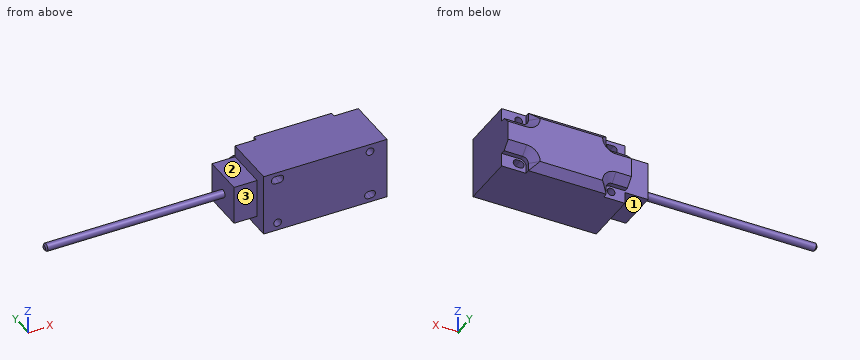
Autodesk Inventor part; units mm, degrees
ref_plane "Work Plane1" through (0, 0, -20) normal (0, 0, 1) x (1, 0, 0)
ref_plane "YZ Plane" through (0, 0, 0) normal (1, 0, 0) x (0, 1, 0)
ref_plane "XZ Plane" through (0, 0, 0) normal (0, 1, 0) x (-1, 0, 0)
sketch "Sketch1" plane through (0, 0, 0) normal (0, 0, 1) x (1, 0, 0)
  line L0 (0, 0) -> (80, 0)
  line L1 (80, 0) -> (80, 43)
  line L2 (80, 43) -> (0, 43)
  line L3 (0, 43) -> (0, 0)
  dimension "d0" = 80
  dimension "d1" = 43
extrude "Extrusion1" add sketch "Sketch1" against normal blind 40
sketch "Sketch2" plane through (0, 43, 0) normal (0, 1, 0) x (1, 0, 0)
  line L0 (80, 0) -> (80, 40)
  circle A0 centre (69, 5) radius 2.5
  arc A1 (7.5, 7.5) -> (7.5, 2.5) centre (7.5, 5) ccw
  arc A2 (10.5, 2.5) -> (10.5, 7.5) centre (10.5, 5) ccw
  line L1 (7.5, 7.5) -> (10.5, 7.5)
  line L2 (10.5, 2.5) -> (7.5, 2.5)
  arc A3 (68, 37.5) -> (68, 32.5) centre (68, 35) ccw
  arc A4 (69.5, 32.5505) -> (70, 37.5) centre (70, 35) ccw
  line L3 (68, 37.5) -> (70, 37.5)
  line L4 (68, 32.5) -> (70, 32.5)
  point P0 (0, 0)
  point P1 (69, 35)
  point P2 (9, 5)
  point P3 (9, 35)
  dimension "d4" = 11
  dimension "d5" = 30
  dimension "d6" = 5
  dimension "d7" = 60
  dimension "d16" = 5
  dimension "d17" = 5
  dimension "d18" = 5
  dimension "d19" = 1.5
  dimension "d20" = 1.5
  dimension "d24" = 5
  dimension "d25" = 5
hole "Hole1" at (69, 43, -5) at (9, 43, -35) direction (0, -1, 0) diameter 5 end through all
extrude "Extrusion2" cut sketch "Sketch2" against normal through all contours L1 A2 L2 A1 | L3 A4 L4 A3
sketch "Sketch3" plane through (0, 43, 0) normal (0, 1, 0) x (1, 0, 0)
  arc A0 (64.25, 35) -> (68, 31.25) centre (68, 35) ccw
  line L0 (64.25, 35) -> (64.25, 40)
  line L1 (68, 31.25) -> (80, 31.25)
  line L2 (64.25, 40) -> (80, 40)
  line L3 (80, 40) -> (80, 31.25)
  line L4 (80, 0) -> (80, 40)
  arc A1 (13.75, 5) -> (10, 8.75) centre (10, 5) ccw
  line L5 (10, 8.75) -> (0, 8.75)
  line L6 (13.75, 5) -> (13.75, 0)
  line L7 (0, 0) -> (80, 0)
  line L8 (0, 0) -> (0, 40)
  line L9 (0, 8.75) -> (0, 0)
  line L10 (0, 0) -> (13.75, 0)
  point P0 (9, 5)
  point P1 (69, 5)
  point P2 (69, 35)
  dimension "d29" = 7.5
  dimension "d34" = 7.5
  dimension "d35" = 1
extrude "Extrusion3" cut sketch "Sketch3" against normal blind 8
ref_plane "Work Plane1" through (0, 0, -20) normal (0, 0, 1) x (1, 0, 0)
mirror "Mirror2" about plane through (0, 0, -20) normal (0, 0, 1) of "Extrusion3"
chamfer "Chamfer1" distance 5 angle 45 14 edges at (39, 43, 0) (39, 43, -40) (5, 43, -8.75) (12.6517, 43, -7.6517) (13.75, 43, -2.5) (12.6517, 43, -32.3483) (5, 43, -31.25) (13.75, 43, -37.5) (74, 43, -31.25) (65.3483, 43, -32.3483) (64.25, 43, -37.5) (74, 43, -8.75) (65.3483, 43, -7.6517) (64.25, 43, -2.5)
sketch "Sketch4" plane through (0, 0, -40) normal (-1, 0, 0) x (0, 0, 1)
  line L0 (7.5, 35) -> (2.5, 35)
  line L1 (7.5, 35) -> (32.5, 35)
  line L2 (32.5, 35) -> (32.5, 8.0021)
  line L3 (32.5, 8.0021) -> (7.5, 8.0021)
  line L4 (7.5, 8.0021) -> (7.5, 35)
  line L5 (7.5, 35) -> (2.5, 35)
  point P0 (40, 0)
extrude "Extrusion4" add sketch "Sketch4" along normal blind 15
sketch "Sketch5" plane through (-15, 0, -40) normal (-1, 0, 0) x (0, 0, 1)
  line L0 (32.5, 35) -> (7.5, 35)
  line L1 (32.5, 8.0021) -> (32.5, 35)
  circle A0 centre (20, 21.5011) radius 2.5
  point P0 (40, 0)
  point P1 (20, 35)
  point P2 (32.5, 21.5011)
  dimension "d41" = 5
extrude "Extrusion5" add sketch "Sketch5" along normal blind 116
chamfer "Chamfer2" distance 1 angle 45 1 edges at (-131, 21.5011, -22.5)
thread "Thread1"
properties part number "802K-MSRS11E" material "ABS Plastic"
The model under review builds one solid part; all positions refer to its coordinate system, in mm. Face numbers are marked on the shaded views. A direction names the side the tool comes from. Coordinates: 2 decimals unless noted, no trailing zeros. Write each loop counter-clockwise with the first axis right and the second up, starting at its lowest first coordinate (ties: lowest second). Pieces come first, ordered by that corner, then holes. Notation, with made-up numbers: (69.5, 62.25) -> (103.5, 62.25) arc R15 cw to (103.5, 87.25) -> close; hole circle Ø8 at (-34.5, 80). An arc over 180 degrees is marked (long way). Answer in a Markdown table with one row per item.
1. We need section D-D, the plane x = -95.5. State the section outline as (y, z) points.
Answers below:
| item | result |
|---|---|
| outline | circle Ø5 at (21.5, -20) |
2. We need section C-C, the plane y = 4. State the section outline as (x, z) points.
Answers below:
| item | result |
|---|---|
| outline | (0, -40) -> (80, -40) -> (80, 0) -> (0, 0) -> close; hole circle Ø5 at (9, -35); hole (7.5, -7.5) -> (10.5, -7.5) arc R2.5 ccw to (10.5, -2.5) -> (7.5, -2.5) arc R2.5 ccw to start; hole circle Ø5 at (69, -5); hole (68, -37.5) -> (70, -37.5) arc R2.5 ccw to (70, -32.5) -> (68, -32.5) arc R2.5 ccw to start |
3. We need section A-A, the plane y = 16.5. State the section outline as (x, z) points.
Answers below:
| item | result |
|---|---|
| outline | (-15, -32.5) -> (0, -32.5) -> (0, -40) -> (80, -40) -> (80, 0) -> (0, 0) -> (0, -7.5) -> (-15, -7.5) -> close; hole circle Ø5 at (9, -35); hole (7.5, -7.5) -> (10.5, -7.5) arc R2.5 ccw to (10.5, -2.5) -> (7.5, -2.5) arc R2.5 ccw to start; hole circle Ø5 at (69, -5); hole (68, -37.5) -> (70, -37.5) arc R2.5 ccw to (70, -32.5) -> (68, -32.5) arc R2.5 ccw to start |
4. Clearance check with flat-ended pins moving along their axes: pin 1 Ø10 at (x, z) = (-50.5, -12) entering from +Y; pin 2 Ø10 at (x, y) = (-109.5, 20.5) entering from +Z; pin 3 Ø2.5 at (x, y) = (71, 36.5) entering from -Z; pin 4 Ø17.5 at (y, z) = (13, -13) entering from -X. State where each tip first meets the part, or that it passes through.
Answers below:
| item | result |
|---|---|
| pin 1 | passes through |
| pin 2 | stops at z = -17.5 |
| pin 3 | stops at z = -31.25 |
| pin 4 | stops at x = -130.24 |
5. Wall thickness on probe 1 along Z at (x, y) = (9, 8); probe 2 along X at (y, z) = (22, -5); probe 3 along X at (y, z) = (22, -29.5): over which ranges is each line inside the solid? List them lowest first. Write a range as [from, to].
Answers below:
| item | result |
|---|---|
| probe 1 | z = [-40, -37.5], [-32.5, -7.5], [-2.5, 0] |
| probe 2 | x = [0, 5], [13, 66.5], [71.5, 80] |
| probe 3 | x = [-15, 80] |
6. We need section B-B, the plane x = -9. State the section outline as (y, z) points, and give its area (3 significant figures).
Answers below:
| item | result |
|---|---|
| outline | (8, -32.5) -> (35, -32.5) -> (35, -7.5) -> (8, -7.5) -> close |
| area | 675 mm^2 |
7. For the marked faces 1, 2 and 3, list the 3-axis set-ups (+Z, -Z, +X, -X, +Y, -Y) from which the entire face can be reached by the end or side of a thin tool; tool diameter is ignored.
Answers below:
| item | result |
|---|---|
| face 1 | -Z, -X, +Y, -Y |
| face 2 | +Z, -X, +Y, -Y |
| face 3 | +Z, -Z, -X, -Y |
